Can you work these out from the model? Positions are in its coordinate system, mm. Face numbers are marked on the shaded views. Round coordinates to 2 decimals unless told otherwise and drop trailing zeros. Write each loop counter-clockwise with the first axis right and the second up, starting at its lowest first coordinate (ties: lowest second). Pieces come first, ordered by that corner, then holes. Notation, with made-up numbers: M 23,84.5 L 27,84.5 A7 ccw 27,94.5 Z; hole C 57,40.5 d2. An arc over 180 degrees is marked long. Answer as a JSON object with one key per item and string values. Group by question number.
1) Please list where these lines run through material, in increasing order: L1, parallel to Z at x = 1.5, y = 4.35; L2, parallel to Z at x = 0.75, y = 1.25; L3, parallel to X at y = -0.3, z = -1.75. Write a range as [from, to].
2) Suppose I cut it at B-B, the plane y = 4.2. Write out the boundary of the cut face in (x, z).
3) If we mould it in two halves opening along X, with no side actions, what happens to the marked faces 1, 2 and 3? For each: +X half, -X half, draft (parallel to the pull), parting line (faces both ways), or undercut.
4) Suppose I cut it at C-C, the plane y = -0.4. Write out the boundary of the cut face in (x, z), and give its area (3 significant figures).
5) I'm going to push flat-ended pins straight in: pin 1 Ø0.7 at (x, z) = (0, -4.5) entering from -Y; pin 2 Ø0.7 at (x, z) = (-1, 4.5) entering from -Y; pin 3 Ø1 at (x, y) = (1, 1.5) entering from +Z; pin 4 Ø2.5 at (x, z) = (0, 0) entering from +Y. Where does each tip first touch, or does it pass through?
6) Suppose I cut it at A-A, the plane y = 2.25. Write out the boundary of the cut face in (x, z).
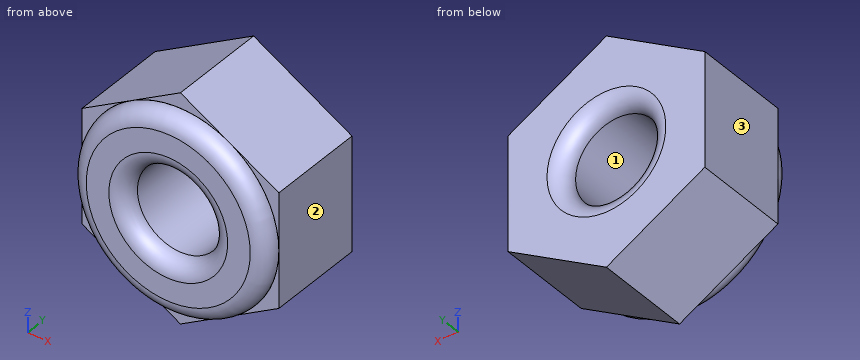
from build123d import *

# Parameters (mm, degrees)
F0_R     = 2.0828
F1_DEPTH = 4.7625
F2_R     = 4.7625
F2_R_2   = 2.0828
F3_DEPTH = 0.79375
F4_R     = 0.79374
F5_R     = 0.79375


# Not quite as in the source:
# - a fillet or chamfer is up to 0.001 mm smaller than in the source, because OpenCascade refuses the exact size


with BuildPart() as f1:
    # F0 (on Front) → F1 (new body)
    with BuildSketch(Plane.XZ):
        Polygon((4.7625, -2.749630657), (4.7625, 2.749630657), (0, 5.499261314), (-4.7625, 2.749630657), (-4.7625, -2.749630657), (0, -5.499261314), align=None)
        Circle(F0_R, mode=Mode.SUBTRACT)
    extrude(amount=-F1_DEPTH)

    # F2 (on face) → F3 (join)
    with BuildSketch(Plane.XZ):
        Circle(F2_R)
        Circle(F2_R_2, mode=Mode.SUBTRACT)
    extrude(amount=F3_DEPTH)

    # F4 (radius 0.79375 in the source; OpenCascade refuses exactly that, so slightly less here)
    f4_edges = [f1.edges().sort_by_distance(p)[0] for p in [
        (-4.7625, -0.79375, 0),
        (-2.0828, -0.79375, 0),
    ]]
    fillet(f4_edges, radius=F4_R)

    # F5
    f5_edges = [f1.edges().sort_by_distance(p)[0] for p in [
        (-2.0828, 4.7625, 0),
    ]]
    fillet(f5_edges, radius=F5_R)


solid = f1.part
Results:
{
 "1": {"L1": "[-4.63, -1.58], [1.58, 4.63]", "L2": "[-5.07, -1.94], [1.94, 5.07]", "L3": "[-4.37, -1.23], [1.23, 4.37]"},
 "2": {"outline": "M -4.76,-2.75 L 0,-5.5 L 4.76,-2.75 L 4.76,2.75 L 0,5.5 L -4.76,2.75 Z; hole C 0,0 d4.23"},
 "3": {"face 1": "undercut", "face 2": "+X half", "face 3": "-X half"},
 "4": {"outline": "C 0,0 d9.31; hole C 0,0 d4.38", "area": "53.0 mm^2"},
 "5": {"pin 1": "y = -0.77", "pin 2": "y = -0.74", "pin 3": "z = 5.21", "pin 4": "through"},
 "6": {"outline": "M -4.76,-2.75 L 0,-5.5 L 4.76,-2.75 L 4.76,2.75 L 0,5.5 L -4.76,2.75 Z; hole C 0,0 d4.17"}
}
